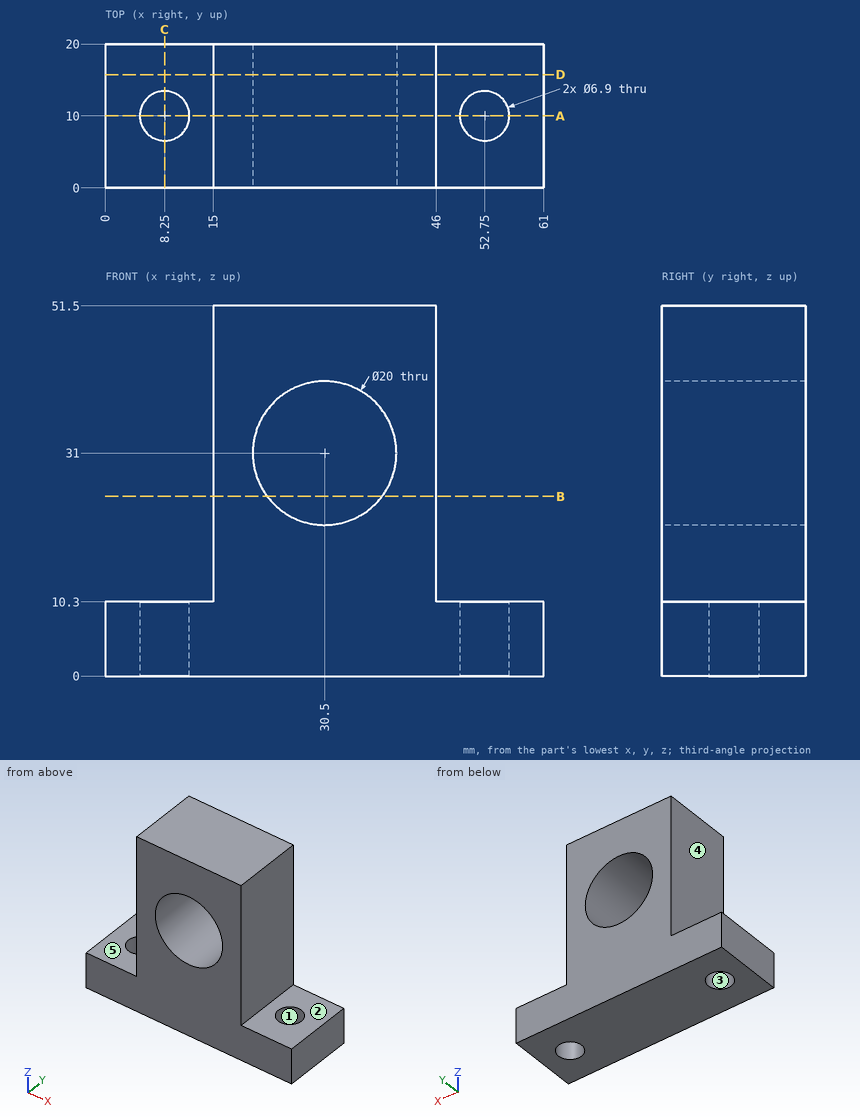
Design review of the part shown in the three views and the two pictorial views. Dimensions are in mm from the part's minimum x, y and z. A direction names the side the tool comes from. Give positions to 0.01 mm unless a question says otherwise; leave off trailing zeros. Write each loop counter-clockwise with the first axis right and the second up, starting at its lowest first coordinate (ties: lowest second). Pieces come first, ordered by that corner, then holes.
(1) Mouldability with a two-part tool opening along X and no side actions: class the marked faces 3, 4 and 5 as +X half, -X half, draft (parallel to the pull), parting line (faces both ways), or undercut.
Checked values:
face 3: undercut
face 4: -X half
face 5: draft
(2) Wall thickness on line 1 along Z through (x, y) = (30.5, 7); line 2 along X through (y, z) = (8.5, 7.5); line 3 along Y through (x, z) = (52.75, 4.5): over which ranges is each line inside the solid? List them lowest first.
Checked values:
line 1: z = 0 to 21, 41 to 51.5
line 2: x = 0 to 5.14, 11.36 to 49.64, 55.86 to 61
line 3: y = 0 to 6.55, 13.45 to 20
(3) Add section B-B (z = 25). Give the boundary of the cut face in (x, y).
Checked values:
outline: (15, 0) - (22.5, 0) - (22.5, 20) - (15, 20) - close; (38.5, 0) - (46, 0) - (46, 20) - (38.5, 20) - close
(4) Tool access review of the marked faces 1 and 2: name each direction out of +Z, -Z, +X, -X, +Y, -Y from which nothing blocks a thin tool from reaching the whole face with its end or side.
Checked values:
face 1: +Z, -Z
face 2: +Z, +X, +Y, -Y
(5) Add section A-A (y = 10). Give the boundary of the cut face in (x, z), and give its area (3 significant figures).
Checked values:
outline: (0, 0) - (4.8, 0) - (4.8, 10.3) - (0, 10.3) - close; (11.7, 0) - (49.3, 0) - (49.3, 10.3) - (46, 10.3) - (46, 51.5) - (15, 51.5) - (15, 10.3) - (11.7, 10.3) - close; (56.2, 0) - (61, 0) - (61, 10.3) - (56.2, 10.3) - close; hole circle Ø20 at (30.5, 31)
area: 1,450 mm2
(6) Add section D-D (y = 15.75). Give the boundary of the cut face in (x, z), and give its area (3 significant figures).
Checked values:
outline: (0, 0) - (61, 0) - (61, 10.3) - (46, 10.3) - (46, 51.5) - (15, 51.5) - (15, 10.3) - (0, 10.3) - close; hole circle Ø20 at (30.5, 31)
area: 1,590 mm2
(7) Clearance check with flat-ended pins moving along their axes: pin 1 Ø8 at (y, z) = (13.5, 13.5) entering from -X; pin 2 Ø6 at (y, z) = (11, 37) entering from +X; pin 3 Ø12 at (x, y) = (54.5, 10.5) entering from +Z; pin 4 Ø10 at (y, z) = (14, 34.5) entering from -X. State where each tip first meets the part, or that it passes through.
Checked values:
pin 1: stops at x = 0
pin 2: stops at x = 46
pin 3: stops at z = 10.3
pin 4: stops at x = 15
(8) Add section C-C (x = 8.25). Give the boundary of the cut face in (y, z).
Checked values:
outline: (0, 0) - (6.55, 0) - (6.55, 10.3) - (0, 10.3) - close; (13.45, 0) - (20, 0) - (20, 10.3) - (13.45, 10.3) - close
